from build123d import *

# Parameters (mm, degrees)
EXTRUDE_1_DEPTH     = 10
SKETCH_2_R          = 1.75
CUT_EXTRUDE_1_DEPTH = 13.5


with BuildPart() as part:
    # ｽｹｯﾁ1 → ﾎﾞｽ - 押し出し1 (new body)
    with BuildSketch(Plane.XY):
        Polygon((0, 0), (0, 9.5), (-5, 9.5), (-5, 12.5), (8, 12.5), (8, 0), align=None)
    extrude(amount=EXTRUDE_1_DEPTH)

    # ｽｹｯﾁ2 → ｶｯﾄ - 押し出し1 (cut, through all)
    with BuildSketch(Plane.XZ):
        with Locations((4, 5)):
            Circle(SKETCH_2_R)
    extrude(amount=-CUT_EXTRUDE_1_DEPTH, mode=Mode.SUBTRACT)


solid = part.part
Input: part model. Units: mm. Frame: model coordinates. A direction names the side the tool comes from. Coordinates: 2 decimals unless noted, no trailing zeros. Loops run counter-clockwise (first coordinate to the right, second up) from the corner with the lowest first, then second, coordinate; pieces in that order, holes last.
(1) Material intervals for probe 1 along Z at (x, y) = (4, 6); probe 2 along X at (y, z) = (6.25, 1.25); probe 3 along Z at (x, y) = (3, 6), sorted ascending.
(2) Section A-A on x = 4. Return the cut outline in (y, z), then the cut area to 4 significant figures.
(3) First-contact query: pin 1 Ø4 at (x, z) = (-3.5, 5) entering from -Y; pin 2 Ø3 at (y, z) = (3, 4) entering from -X. Flat tips, straight axial feed; report the tip coordinate or a pass-through.
(4) Section B-B on z = 5. Return the cut outline in (x, y), then the cut area to 4 significant figures.
(5) Section D-D on x = -2.75. Return the cut outline in (y, z), then the cut area to 3 significant figures.
(6) Section C-C on y = 11.75. Return the cut outline in (x, z), then the cut area to 3 significant figures.
(7) Pull-direction query (X, two-part tool) for faces 1 (the face through (2.61, 6.16, 3.94)), 2 (the face through (8, 6, 5)), 3 (the face through (3, 6, 10)), 4 (the face through (-5, 11, 5)); classes: released by +X, released by -X, zero draft, split by the parting line, or undercut.
(8) Set-up query: faces 5 (the face through (1, 12.5, 5)), 6 (the face through (0, 5, 5)). Return all of +Z, -Z, +X, -X, +Y, -Y with unobstructed straight access to the full face (end or side cutting, diameter ignored); none if empty.
Data:
1. probe 1: z = 0 to 3.25, 6.75 to 10
1. probe 2: x = 0 to 8
1. probe 3: z = 0 to 3.56, 6.44 to 10
2. outline: (0, 0) - (12.5, 0) - (12.5, 3.25) - (0, 3.25) - close; (0, 6.75) - (12.5, 6.75) - (12.5, 10) - (0, 10) - close
2. area: 81.25 mm2
3. pin 1: stops at y = 9.5
3. pin 2: stops at x = 0
4. outline: (-5, 9.5) - (0, 9.5) - (0, 0) - (2.25, 0) - (2.25, 12.5) - (-5, 12.5) - close; (5.75, 0) - (8, 0) - (8, 12.5) - (5.75, 12.5) - close
4. area: 71.25 mm2
5. outline: (9.5, 0) - (12.5, 0) - (12.5, 10) - (9.5, 10) - close
5. area: 30.0 mm2
6. outline: (-5, 0) - (8, 0) - (8, 10) - (-5, 10) - close; hole circle Ø3.5 at (4, 5)
6. area: 120 mm2
7. face 1: undercut
7. face 2: released by +X
7. face 3: zero draft
7. face 4: released by -X
8. face 5: +Z, -Z, +X, -X, +Y
8. face 6: +Z, -Z, -X, -Y
